Input: part model. Units: mm. Frame: model coordinates. Coordinates: 2 decimals unless noted, no trailing zeros. Write each loop counter-clockwise with the first axis right and the second up, starting at its lowest first coordinate (ties: lowest second). Pieces come first, ordered by that corner, then holes. Notation, with made-up numbers: (35, 26.25) -> (49, 26.25) arc R18 cw to (49, 35.25) -> close; hole circle Ø9 at (9.25, -10.5). An arc over 180 degrees is marked (long way). Use one line per item in the form item = value. Start each with the question number.
(1) Cut plane C-C on x = -80.5. Return the cut outline in (y, z), plus the area to 3 significant figures.
(2) Cut plane B-B on x = -50. Return the cut outline in (y, z).
(3) First-contact query: pin 1 (3 mm diameter, centred on x = -81.5, z = 1, fed in from +Y); pin 2 (1.8 mm diameter, centred on y = 37, z = 4, fed in from -X); pin 3 (3 mm diameter, centred on y = 142, z = 3, fed in from +X). Flat tips, straight axial feed; report the tip coordinate or a pass-through.
(4) Cut plane A-A on y = 154.5. Return the cut outline in (x, z), plus the area to 3 significant figures.
(5) Cut plane D-D on x = -173. Return the cut outline in (y, z).
(6) Ray query, line 1 along X through (y, z) = (151.5, 2.35); line 2 along X through (y, z) = (131.5, 5.15); line 3 along Y through (x, z) = (-50, 3). Return the intervals inside material, ascending.
```python
from build123d import *

# Parameters (mm, degrees)
BOSS_EXTRUDE1_DEPTH   = 6
SKETCH2_W             = 6
SKETCH2_H             = 25
BOSS_EXTRUDE2_DEPTH   = 6
LPATTERN1_OUTLINE_W   = 6
LPATTERN1_OUTLINE_H   = 6
LPATTERN1_DEPTH       = 25
LPATTERN1_START       = 50
LPATTERN1_2_OUTLINE_W = 6
LPATTERN1_2_OUTLINE_H = 6
LPATTERN1_2_DEPTH     = 25
LPATTERN1_START_2     = 100
LPATTERN1_3_OUTLINE_W = 6
LPATTERN1_3_OUTLINE_H = 6
LPATTERN1_3_DEPTH     = 25
LPATTERN1_START_3     = 150
LPATTERN1_4_OUTLINE_W = 6
LPATTERN1_4_OUTLINE_H = 6
LPATTERN1_4_DEPTH     = 25
SKETCH5_R             = 4
CUT_EXTRUDE1_DEPTH    = 271.364568685


# Read off the part's stored shape, not the designer's step: LPattern1
with BuildPart() as part:
    # Sketch1 → Boss-Extrude1 (new body)
    with BuildSketch(Plane.XY):
        with BuildLine():
            Line((-178, 175), (-200, 175))
            Line((-200, 175), (-200, 0))
            Line((-200, 0), (0, 0))
            Line((0, 0), (0, 175))
            Line((0, 175), (-22, 175))
            Line((-22, 175), (-22, 110))
            ThreePointArc((-22, 110), (-31.037807258, 73.555302549), (-56.056819802, 45.55625))
            ThreePointArc((-56.056819802, 45.55625), (-100, 27.5), (-143.943180198, 45.55625))
            ThreePointArc((-143.943180198, 45.55625), (-168.962192742, 73.555302549), (-178, 110))
            Line((-178, 110), (-178, 175))
        make_face()
    extrude(amount=BOSS_EXTRUDE1_DEPTH)

    # Sketch2 → Boss-Extrude2 (add)
    with BuildSketch(Plane.XY.offset(6)):
        with Locations((-203, 162.5)):
            Rectangle(SKETCH2_W, SKETCH2_H)
    extrude(amount=-BOSS_EXTRUDE2_DEPTH)

    # LPattern1 outline → LPattern1 (add)
    with BuildSketch(Plane(origin=(0, 0, 0), x_dir=(1, 0, 0), z_dir=(0, 1, 0))):
        with Locations((-203, -3)):
            Rectangle(LPATTERN1_OUTLINE_W, LPATTERN1_OUTLINE_H)
        with Locations((3, -3)):
            Rectangle(LPATTERN1_OUTLINE_W, LPATTERN1_OUTLINE_H)
    extrude(amount=LPATTERN1_DEPTH)

    # LPattern1 2 outline → LPattern1 2 (add)
    with BuildSketch(Plane(origin=(0, 0, 0), x_dir=(1, 0, 0), z_dir=(0, 1, 0)).offset(LPATTERN1_START)):
        with Locations((-203, -3)):
            Rectangle(LPATTERN1_2_OUTLINE_W, LPATTERN1_2_OUTLINE_H)
        with Locations((3, -3)):
            Rectangle(LPATTERN1_2_OUTLINE_W, LPATTERN1_2_OUTLINE_H)
    extrude(amount=LPATTERN1_2_DEPTH)

    # LPattern1 3 outline → LPattern1 3 (add)
    with BuildSketch(Plane(origin=(0, 0, 0), x_dir=(1, 0, 0), z_dir=(0, 1, 0)).offset(LPATTERN1_START_2)):
        with Locations((-203, -3)):
            Rectangle(LPATTERN1_3_OUTLINE_W, LPATTERN1_3_OUTLINE_H)
        with Locations((3, -3)):
            Rectangle(LPATTERN1_3_OUTLINE_W, LPATTERN1_3_OUTLINE_H)
    extrude(amount=LPATTERN1_3_DEPTH)

    # LPattern1 4 outline → LPattern1 4 (add)
    with BuildSketch(Plane(origin=(0, 0, 0), x_dir=(1, 0, 0), z_dir=(0, 1, 0)).offset(LPATTERN1_START_3)):
        with Locations((3, -3)):
            Rectangle(LPATTERN1_4_OUTLINE_W, LPATTERN1_4_OUTLINE_H)
    extrude(amount=LPATTERN1_4_DEPTH)

    # Sketch5 → Cut-Extrude1 (cut, through all)
    with BuildSketch(Plane.XY.offset(6)):
        with Locations((-50, 25)):
            Circle(SKETCH5_R)
    extrude(amount=-CUT_EXTRUDE1_DEPTH, mode=Mode.SUBTRACT)


solid = part.part
```
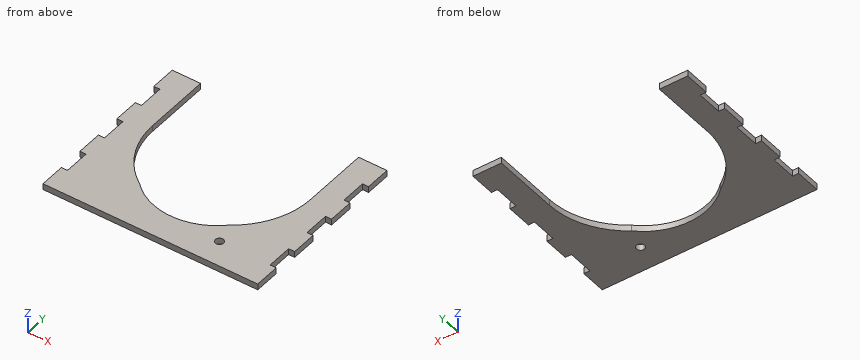
Values:
q1.outline = (0, 0) -> (30.62, 0) -> (30.62, 6) -> (0, 6) -> close
q1.area = 184 mm2
q2.outline = (0, 0) -> (21, 0) -> (21, 6) -> (0, 6) -> close; (29, 0) -> (50.13, 0) -> (50.13, 6) -> (29, 6) -> close
q3.pin_1 = 30.79
q3.pin_2 = -200
q3.pin_3 = 0
q4.outline = (-206, 0) -> (-178, 0) -> (-178, 6) -> (-206, 6) -> close; (-22, 0) -> (6, 0) -> (6, 6) -> (-22, 6) -> close
q4.area = 336 mm2
q5.outline = (0, 0) -> (82.52, 0) -> (82.52, 6) -> (0, 6) -> close
q6.line_1 = -206 to -178, -22 to 6
q6.line_2 = -200 to -178, -22 to 0
q6.line_3 = 0 to 21, 29 to 50.13
